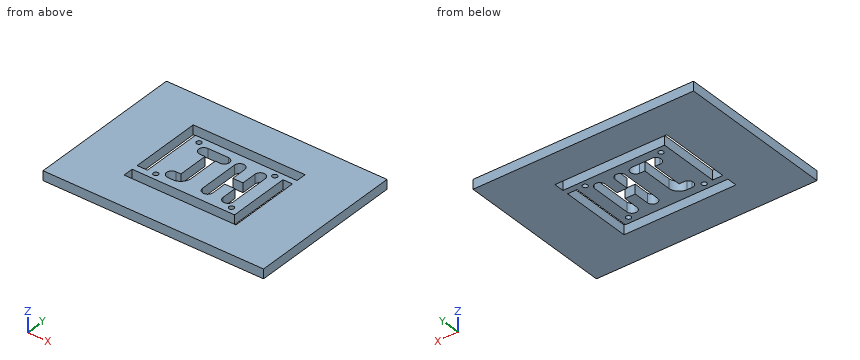
Autodesk Inventor part; units mm, degrees
ref_plane "YZ Plane" through (0, 0, 0) normal (1, 0, 0) x (0, 1, 0)
ref_plane "XZ Plane" through (0, 0, 0) normal (0, 1, 0) x (-1, 0, 0)
ref_plane "XY Plane" through (0, 0, 0) normal (0, 0, 1) x (1, 0, 0)
sketch "Sketch1" plane through (0, 0, 0) normal (0, 0, 1) x (1, 0, 0)
  arc A0 (0, 6.5) -> (0, -6.5) centre (0, 0) ccw
  line L0 (0, 6.5) -> (26, 6.5)
  line L1 (0, -6.5) -> (6.5, -6.5)
  arc A1 (26, -6.5) -> (26, 6.5) centre (26, 0) ccw
  line L2 (26, -6.5) -> (19.5, -6.5)
  line L3 (6.5, -6.5) -> (6.5, -45.5)
  line L4 (19.5, -6.5) -> (19.5, -45.5)
  line L5 (6.5, -45.5) -> (0, -45.5)
  arc A2 (0, -45.5) -> (0, -58.5) centre (0, -52) ccw
  line L6 (0, -58.5) -> (6.5, -58.5)
  arc A3 (6.5, -58.5) -> (19.5, -45.5) centre (6.5, -45.5) ccw
  line L7 (39, 0) -> (39, -52)
  arc A4 (39, -52) -> (52, -52) centre (45.5, -52) ccw
  line L8 (52, -52) -> (52, -32.5)
  line L9 (52, -32.5) -> (65, -32.5)
  line L10 (65, 0) -> (65, -19.5)
  line L11 (65, -19.5) -> (52, -19.5)
  line L12 (52, -19.5) -> (52, 0)
  line L13 (78, 0) -> (78, -52)
  line L14 (65, -32.5) -> (65, -52)
  arc A5 (65, -52) -> (78, -52) centre (71.5, -52) ccw
  arc A6 (52, 0) -> (39, 0) centre (45.5, 0) ccw
  arc A7 (78, 0) -> (65, 0) centre (71.5, 0) ccw
  point P0 (0, 0)
  point P1 (0, 0)
  dimension "d0" = 26
  dimension "d1" = 6.5
  dimension "d2" = 13
  dimension "d3" = 13
  dimension "d4" = 6.5
  dimension "d5" = 13
  dimension "d6" = 39
  dimension "d7" = 39
  dimension "d8" = 6.5
  dimension "d9" = 52
  dimension "d10" = 6.5
  dimension "d11" = 13
  dimension "d12" = 19.5
  dimension "d13" = 13
  dimension "d14" = 13
  dimension "d15" = 13
  dimension "d16" = 19.5
  dimension "d17" = 13
  dimension "d19" = 52
  dimension "d20" = 13
  dimension "d22" = 6.5
  dimension "d23" = 19.5
  dimension "d24" = 6.5
  dimension "d53" = 19.5
sketch "Sketch2" plane through (0, 0, 0) normal (0, 0, 1) x (1, 0, 0)
  circle A0 centre (-13.3188, 9.1594) radius 3.175
  circle A1 centre (-13.3188, -60.8406) radius 3.175
  circle A2 centre (82.6812, -60.8406) radius 3.175
  circle A3 centre (82.6812, 9.4938) radius 3.175
  line L0 (-24, 17) -> (93, 17)
  line L1 (93, 17) -> (93, -69)
  line L2 (93, -69) -> (-24, -69)
  line L3 (-24, -69) -> (-24, 17)
  line L4 (-105.5, 74) -> (174.5, 74)
  line L5 (174.5, 74) -> (174.5, -126)
  line L6 (174.5, -126) -> (-105.5, -126)
  line L7 (-105.5, -126) -> (-105.5, 74)
  line L8 (93, 9.4938) -> (105, 9.4938)
  line L9 (105, 9.4938) -> (105, -69)
  line L10 (105, -69) -> (93, -69)
  line L11 (93, -69) -> (93, 9.4938)
  line L12 (-24, -69) -> (105, -69)
  line L13 (-24, 17) -> (-24, -60.8406)
  line L14 (105, -82) -> (-37, -82)
  line L15 (-37, -82) -> (-37, -69)
  line L16 (-37, -69) -> (105, -69)
  line L17 (105, -69) -> (105, -82)
  line L18 (-24, -60.8406) -> (-37, -60.8406)
  line L19 (-37, -60.8406) -> (-37, 30)
  line L20 (-37, 30) -> (-24, 30)
  line L21 (-24, 30) -> (-24, -60.8406)
  line L22 (-24, 17) -> (105, 17)
  line L23 (105, 17) -> (105, 30)
  line L24 (105, 30) -> (-24, 30)
  line L25 (-24, 30) -> (-24, 17)
  point P0 (0, 0)
  point P1 (82.6812, 17)
  dimension "d54" = 6.35
  dimension "d55" = 6.35
  dimension "d56" = 6.35
  dimension "d57" = 6.35
  dimension "d62" = 117
  dimension "d63" = 86
  dimension "d64" = 280
  dimension "d65" = 200
  dimension "d66" = 57
  dimension "d68" = 17
  dimension "d69" = 24
  dimension "d70" = 81.5
extrude "Extrusion6" add sketch "Sketch2" against normal blind 12 contours L0 L1 L2 L3 | L4 L5 L6 L7
extrude "Extrusion7" cut sketch "Sketch1" against normal blind 12
properties part number "JH" material "Polyethylene, High Density"
Could you check a few things on this model? Use its own coordinates, in mm. Round coordinates to 2 decimals unless told otherwise and drop trailing zeros. Order: outer loops, then holes, each group sorted by start corner. A loop starts at its lowest first (then second) coordinate and runs counter-clockwise, first axis right, second up.
Q1. Imagine slicing it at B-B, the plane x = 99. List the corners of the cut face in (y, z) for me.
Geometry says:
outline: (-126, -12) - (-82, -12) - (-82, 0) - (-126, 0) - close; (9.49, -12) - (17, -12) - (17, 0) - (9.49, 0) - close; (30, -12) - (74, -12) - (74, 0) - (30, 0) - close
Q2. Imagine slicing it at D-D, the plane z = -4.5. State how many separate pieces and enclosed holes the cut face has, then the cut area to 3 significant figures.
Geometry says:
separate pieces: 1
enclosed holes: 8
area: 47,200 mm2
Q3. Imagine slicing it at C-C, the plane x = 10. List the corners of the cut face in (y, z) for me.
Geometry says:
outline: (-126, -12) - (-82, -12) - (-82, 0) - (-126, 0) - close; (-69, -12) - (-58.02, -12) - (-58.02, 0) - (-69, 0) - close; (6.5, -12) - (17, -12) - (17, 0) - (6.5, 0) - close; (30, -12) - (74, -12) - (74, 0) - (30, 0) - close
Q4. Imagine slicing it at A-A, the plane x = 45.5. List the corners of the cut face in (y, z) for me, then the cut area to 3 significant figures.
Geometry says:
outline: (-126, -12) - (-82, -12) - (-82, 0) - (-126, 0) - close; (-69, -12) - (-58.5, -12) - (-58.5, 0) - (-69, 0) - close; (6.5, -12) - (17, -12) - (17, 0) - (6.5, 0) - close; (30, -12) - (74, -12) - (74, 0) - (30, 0) - close
area: 1,310 mm2
Q5. Please list where these lines run through material, in increasing order: probe 1 along X at (y, z) = (-44, -6.5); probe 2 along Y at (x, z) = (-21.5, -9.75); probe 3 along Y at (x, z) = (59.5, -8.25).
Geometry says:
probe 1: x = -105.5 to -37, -24 to 6.5, 19.5 to 39, 52 to 65, 78 to 93, 105 to 174.5
probe 2: y = -126 to -82, -69 to 17, 30 to 74
probe 3: y = -126 to -82, -69 to -32.5, -19.5 to 17, 30 to 74
Q6. I'm going to push a flat-ended pin straight in: P1, Ø5, axis at x = -26.5, y = -72.5, coming from the -Z side. Where does the tip first touch, or does it pass through?
Geometry says:
P1: passes through
